Geometry: final body of the model. Coordinates: model frame, mm. A direction names the side the tool comes from. Round coordinates to 2 decimals unless told otherwise and drop trailing zeros. Order: outer loops, then holes, each group sorted by start corner. A loop starts at its lowest first (then second) coordinate and runs counter-clockwise, first axis right, second up. Notation, with made-up numbers: (70, 46) -> (75, 46) arc R4 cw to (75, 51) -> close; hole circle Ø7 at (81, 23). An arc over 180 degrees is marked (long way). Put each result on its own line as item: value.
```python
from build123d import *

# Parameters (mm, degrees)
SKETCH1_R           = 14.641801201
BOSS_EXTRUDE1_DEPTH = 4
SKETCH2_R           = 2
CUT_EXTRUDE1_DEPTH  = 16
SKETCH3_W           = 17
SKETCH3_H           = 16
CUT_EXTRUDE2_DEPTH  = 7


with BuildPart() as part:
    # Sketch1 → Boss-Extrude1 (new body)
    with BuildSketch(Plane(origin=(0, 0, 0), x_dir=(-1, 0, 0), z_dir=(0, 0, 1))):
        with BuildLine():
            Line((8.946512726, 42.193608765), (-46.053487274, 42.193608765))
            Line((-46.053487274, 42.193608765), (-46.053487274, 114.193608765))
            Line((-46.053487274, 114.193608765), (55.263162893, 114.193608765))
            Line((55.263162893, 114.193608765), (55.263162893, 24.601563698))
            Line((55.263162893, 24.601563698), (16.538557793, 24.601563698))
            ThreePointArc((16.538557793, 24.601563698), (11.170171243, 26.825222215), (8.946512726, 32.193608765))
            Line((8.946512726, 32.193608765), (8.946512726, 42.193608765))
        make_face()
        with Locations(Location((34.486512726, 47.671563698, 0), (0, 0, 180))):
            Circle(SKETCH1_R, mode=Mode.SUBTRACT)
    extrude(amount=BOSS_EXTRUDE1_DEPTH)

    # Sketch2 → Cut-Extrude1 (cut)
    with BuildSketch(Plane.XY.offset(4)):
        with Locations((41.553487274, -109.693608765)):
            Circle(SKETCH2_R)
        with Locations((31.553487274, -109.693608765)):
            Circle(SKETCH2_R)
        with Locations((-50.763162893, -109.693608765)):
            Circle(SKETCH2_R)
        with Locations((-40.763162893, -109.693608765)):
            Circle(SKETCH2_R)
        with Locations((41.553487274, -64.693608765)):
            Circle(SKETCH2_R)
        with Locations((31.553487274, -64.693608765)):
            Circle(SKETCH2_R)
        with Locations((-4.446512726, -64.693608765)):
            Circle(SKETCH2_R)
        with Locations((5.553487274, -64.693608765)):
            Circle(SKETCH2_R)
    extrude(amount=-CUT_EXTRUDE1_DEPTH, mode=Mode.SUBTRACT)

    # Sketch3 → Cut-Extrude2 (cut)
    with BuildSketch(Plane.XY.offset(4)):
        with Locations((18.553487274, -60.193608765)):
            Rectangle(SKETCH3_W, SKETCH3_H)
    extrude(amount=-CUT_EXTRUDE2_DEPTH, mode=Mode.SUBTRACT)


solid = part.part
```
1. Cut plane B-B on y = -36. Return loops of the section in (x, z), and give its area (3 significant figures).
Ans:
outline: (-55.26, 0) -> (-43.33, 0) -> (-43.33, 4) -> (-55.26, 4) -> close; (-25.65, 0) -> (-8.95, 0) -> (-8.95, 4) -> (-25.65, 4) -> close
area: 115 mm²
2. Material intervals for probe 1 along Y at (x, z) = (14.5, 3.1); probe 2 along X at (y, z) = (-59, 2.05); probe 3 along X at (y, z) = (-40, 3.35), sorted ascending.
Ans:
probe 1: -114.19 to -68.19, -52.19 to -42.19
probe 2: -55.26 to -43.76, -25.21 to 10.05, 27.05 to 46.05
probe 3: -55.26 to -46.96, -22.02 to -8.95
3. Draft query along X for faces 4 (the face through (46.053, -78, 2)), 5 (the face through (5.29, -62.71, 2.03)), 6 (the face through (-55.263, -70, 2)). Return one class per face: +X half, -X half, draft (parallel to the pull), parting line (faces both ways), or undercut.
Ans:
face 4: +X half
face 5: undercut
face 6: -X half
4. Set-up query: faces 1 (the face through (-4, -114.194, 2)), 2 (the face through (18, -42.194, 2)), 3 (the face through (27.053, -60, 2)). Return all of +Z, -Z, +X, -X, +Y, -Y with unobstructed straight access to the full face (end or side cutting, diameter ignored); none if empty.
Ans:
face 1: +Z, -Z, +X, -X, -Y
face 2: +Z, -Z, +X, +Y
face 3: +Z, -Z
5. Cut plane C-C on z = 1.25. State how many separate pieces and enclosed holes the cut face has, and give its area (3 significant figures).
Ans:
separate pieces: 1
enclosed holes: 10
area: 7,050 mm²
6. Cut plane D-D on y = -54. Return loops of the section in (x, z), and give its area (3 significant figures).
Ans:
outline: (-55.26, 0) -> (-47.69, 0) -> (-47.69, 4) -> (-55.26, 4) -> close; (-21.28, 0) -> (10.05, 0) -> (10.05, 4) -> (-21.28, 4) -> close; (27.05, 0) -> (46.05, 0) -> (46.05, 4) -> (27.05, 4) -> close
area: 232 mm²
7. Cut plane A-A on x = 17. Return loops of the section in (y, z), and give its area (3 significant figures).
Ans:
outline: (-114.19, 0) -> (-68.19, 0) -> (-68.19, 4) -> (-114.19, 4) -> close; (-52.19, 0) -> (-42.19, 0) -> (-42.19, 4) -> (-52.19, 4) -> close
area: 224 mm²
8. Contact query for a flat-ended pin moving along its axis: P1, Ø2, axis at x = 22.5, z = 2, coming from the +Y side. Output: stop coordinate, or through.
Ans:
P1: y = -42.19
